```python
from build123d import *

# Parameters (mm, degrees)
SKETCH1_R           = 1.65
SKETCH1_R_2         = 10.5
BOSS_EXTRUDE1_DEPTH = 3


with BuildPart() as part:
    # Sketch1 → Boss-Extrude1 (new body)
    with BuildSketch(Plane.XY):
        with BuildLine():
            Line((0, 7.5), (32.95, 7.5))
            ThreePointArc((32.95, 7.5), (40.021067812, 10.428932188), (42.95, 17.5))
            Line((42.95, 17.5), (42.95, 28))
            ThreePointArc((42.95, 28), (58.45, 43.5), (73.95, 28))
            Line((73.95, 28), (73.95, 0))
            ThreePointArc((73.95, 0), (73.692468135, -1.526015624), (72.948398416, -2.883))
            Line((72.948398416, -2.883), (69.3, -7.5))
            Line((69.3, -7.5), (0, -7.5))
            Line((0, -7.5), (-3.648398416, -2.883))
            ThreePointArc((-3.648398416, -2.883), (-4.65, 0), (-3.648398416, 2.883))
            Line((-3.648398416, 2.883), (0, 7.5))
        make_face()
        Circle(SKETCH1_R, mode=Mode.SUBTRACT)
        with Locations((69.3, 0)):
            Circle(SKETCH1_R, mode=Mode.SUBTRACT)
        with Locations((58.45, 28)):
            Circle(SKETCH1_R_2, mode=Mode.SUBTRACT)
    extrude(amount=BOSS_EXTRUDE1_DEPTH)


solid = part.part
```
Here's how the part is built. I have some questions about the finished solid (model axes, mm). A direction names the side the tool comes from. Coordinates: 2 decimals unless noted, no trailing zeros. Order: outer loops, then holes, each group sorted by start corner. A loop starts at its lowest first (then second) coordinate and runs counter-clockwise, first axis right, second up.
Item 1: If we section it at B-B, the plane y = 19.5: List the corners of the cut face in (x, z) for me, then the cut area to 3 significant figures.
Response values:
outline: (42.95, 0) - (52.29, 0) - (52.29, 3) - (42.95, 3) - close; (64.61, 0) - (73.95, 0) - (73.95, 3) - (64.61, 3) - close
area: 56.0 mm2
Item 2: If we section it at D-D, the plane x = 25: List the corners of the cut face in (y, z) for me, then the cut area to 3 significant figures.
Response values:
outline: (-7.5, 0) - (7.5, 0) - (7.5, 3) - (-7.5, 3) - close
area: 45.0 mm2
Item 3: Thinking about a two-plate mould opening in X: for faces 1 (the face through (73.7, -1.5, 1.5)), 2 (the face through (-1.216, 1.115, 1.479)), 3 (the face through (-4.65, -0.04, 1.48)), which applies, pulls with the +X half, pulls with the -X half, needs draft (parallel to the pull), parting line crosses it, or undercut?
Response values:
face 1: pulls with the +X half
face 2: undercut
face 3: pulls with the -X half
Item 4: I need wall thicknesses on probe 1 along Y at (x, z) = (58.45, 2.4); probe 2 along X at (y, z) = (35, 2.3); probe 3 along Y at (x, z) = (54.5, 0.4). Which ranges of each line are inside material? Lowest first, please.
Response values:
probe 1: y = -7.5 to 17.5, 38.5 to 43.5
probe 2: x = 44.62 to 50.62, 66.28 to 72.28
probe 3: y = -7.5 to 18.27, 37.73 to 42.99
Item 5: If we section it at C-C, the plane x = 54: List the corners of the cut face in (y, z) for me, then the cut area to 3 significant figures.
Response values:
outline: (-7.5, 0) - (18.49, 0) - (18.49, 3) - (-7.5, 3) - close; (37.51, 0) - (42.85, 0) - (42.85, 3) - (37.51, 3) - close
area: 94.0 mm2
Item 6: If we section it at A-A, the plane z = 1.85: List the corners of the cut face in (x, y) for me, then the cut area to 3 significant figures.
Response values:
outline: (-3.65, -2.88) - (0, -7.5) - (69.3, -7.5) - (72.95, -2.88) arc R4.65 ccw to (73.95, 0) - (73.95, 28) arc R15.5 ccw to (42.95, 28) - (42.95, 17.5) arc R10 cw to (32.95, 7.5) - (0, 7.5) - (-3.65, 2.88) arc R4.65 ccw to start; hole circle Ø3.3 at (0, 0); hole circle Ø21 at (58.45, 28); hole circle Ø3.3 at (69.3, 0)
area: 1,810 mm2
Item 7: Which directions (+Z, -Z, +X, -X, +Y, -Y) give clear straight access to the entire face, cutting with the end or side of a thin tool? Please do faces 4 (the face through (16, 7.5, 1)), 5 (the face through (-1.8, -5.22, 1.48)).
Response values:
face 4: +Z, -Z, -X, +Y
face 5: +Z, -Z, -X, -Y
Item 8: I'm going to push a flat-ended pin straight in: pin 1 Ø1.5 at (y, z) = (25, 2) entering from -X. Where does the tip first touch, or does it pass through?
Response values:
pin 1: stops at x = 42.95
